```python
from build123d import *

# Parameters (mm, degrees)
EXTRUDE_1_DEPTH                  = 27.5
SKETCH_2_W                       = 5
SKETCH_2_H                       = 21
CUT_EXTRUDE_1_DEPTH              = 3
PATTERN_LINEAR_1_COUNT           = 3
PATTERN_LINEAR_1_PITCH           = 10
PATTERN_LINEAR_2_COPY_1_SKETCH_W = 5
PATTERN_LINEAR_2_COPY_1_SKETCH_H = 21
PATTERN_LINEAR_2_COPY_1_DEPTH    = 3
PATTERN_LINEAR_2_COPY_2_SKETCH_W = 5
PATTERN_LINEAR_2_COPY_2_SKETCH_H = 21
PATTERN_LINEAR_2_COPY_2_DEPTH    = 3
PATTERN_LINEAR_2_COPY_3_SKETCH_W = 5
PATTERN_LINEAR_2_COPY_3_SKETCH_H = 21
PATTERN_LINEAR_2_COPY_3_DEPTH    = 3
PATTERN_LINEAR_2_COPY_4_SKETCH_W = 5
PATTERN_LINEAR_2_COPY_4_SKETCH_H = 21
PATTERN_LINEAR_2_COPY_4_DEPTH    = 3
PATTERN_LINEAR_2_COPY_5_SKETCH_W = 5
PATTERN_LINEAR_2_COPY_5_SKETCH_H = 21
PATTERN_LINEAR_2_COPY_5_DEPTH    = 3
PATTERN_LINEAR_2_COPY_6_SKETCH_W = 5
PATTERN_LINEAR_2_COPY_6_SKETCH_H = 21
PATTERN_LINEAR_2_COPY_6_DEPTH    = 3
CUT_EXTRUDE_2_DEPTH              = 31.504098085
CUT_EXTRUDE_2_DEPTH_BACK         = 55
SKETCH_3_R                       = 2.5
CUT_EXTRUDE_3_DEPTH              = 31.504098085
SKETCH_5_R                       = 4.5
CUT_EXTRUDE_4_DEPTH              = 5.5


with BuildPart() as part:
    # 草图1 → 凸台-拉伸1 (new, symmetric)
    with BuildSketch(Plane(origin=(0, 0, 0), x_dir=(0, 0, -1), z_dir=(1, 0, 0))):
        Polygon((-8, 0), (8, 0), (8, 2.916666667), (10.5, 5), (8, 8), (-8, 8), (-10.5, 5), (-8, 2.916666667), align=None)
    extrude(amount=EXTRUDE_1_DEPTH, both=True)

    # 草图2 → 切除-拉伸1 (cut)
    with BuildSketch(Plane(origin=(0, 8, 0), x_dir=(1, 0, 0), z_dir=(0, 1, 0))):
        Rectangle(SKETCH_2_W, SKETCH_2_H)
    cut_extrude_1 = extrude(amount=-CUT_EXTRUDE_1_DEPTH, mode=Mode.SUBTRACT)

    # 阵列(线性)1: 切除-拉伸1 ×3
    with Locations(*[(i * PATTERN_LINEAR_1_PITCH, 0, 0) for i in range(1, PATTERN_LINEAR_1_COUNT)]):
        add(cut_extrude_1, mode=Mode.SUBTRACT)

    # 阵列(线性)2 copy 1 sketch → 阵列(线性)2 copy 1 (cut)
    with BuildSketch(Plane(origin=(0, 8, 0), x_dir=(1, 0, 0), z_dir=(0, 1, 0))):
        Rectangle(PATTERN_LINEAR_2_COPY_1_SKETCH_W, PATTERN_LINEAR_2_COPY_1_SKETCH_H)
    extrude(amount=-PATTERN_LINEAR_2_COPY_1_DEPTH, mode=Mode.SUBTRACT)

    # 阵列(线性)2 copy 2 sketch → 阵列(线性)2 copy 2 (cut)
    with BuildSketch(Plane(origin=(-10, 8, 0), x_dir=(1, 0, 0), z_dir=(0, 1, 0))):
        Rectangle(PATTERN_LINEAR_2_COPY_2_SKETCH_W, PATTERN_LINEAR_2_COPY_2_SKETCH_H)
    extrude(amount=-PATTERN_LINEAR_2_COPY_2_DEPTH, mode=Mode.SUBTRACT)

    # 阵列(线性)2 copy 3 sketch → 阵列(线性)2 copy 3 (cut)
    with BuildSketch(Plane(origin=(10, 8, 0), x_dir=(1, 0, 0), z_dir=(0, 1, 0))):
        Rectangle(PATTERN_LINEAR_2_COPY_3_SKETCH_W, PATTERN_LINEAR_2_COPY_3_SKETCH_H)
    extrude(amount=-PATTERN_LINEAR_2_COPY_3_DEPTH, mode=Mode.SUBTRACT)

    # 阵列(线性)2 copy 4 sketch → 阵列(线性)2 copy 4 (cut)
    with BuildSketch(Plane(origin=(0, 8, 0), x_dir=(1, 0, 0), z_dir=(0, 1, 0))):
        Rectangle(PATTERN_LINEAR_2_COPY_4_SKETCH_W, PATTERN_LINEAR_2_COPY_4_SKETCH_H)
    extrude(amount=-PATTERN_LINEAR_2_COPY_4_DEPTH, mode=Mode.SUBTRACT)

    # 阵列(线性)2 copy 5 sketch → 阵列(线性)2 copy 5 (cut)
    with BuildSketch(Plane(origin=(-10, 8, 0), x_dir=(1, 0, 0), z_dir=(0, 1, 0))):
        Rectangle(PATTERN_LINEAR_2_COPY_5_SKETCH_W, PATTERN_LINEAR_2_COPY_5_SKETCH_H)
    extrude(amount=-PATTERN_LINEAR_2_COPY_5_DEPTH, mode=Mode.SUBTRACT)

    # 阵列(线性)2 copy 6 sketch → 阵列(线性)2 copy 6 (cut)
    with BuildSketch(Plane(origin=(-20, 8, 0), x_dir=(1, 0, 0), z_dir=(0, 1, 0))):
        Rectangle(PATTERN_LINEAR_2_COPY_6_SKETCH_W, PATTERN_LINEAR_2_COPY_6_SKETCH_H)
    extrude(amount=-PATTERN_LINEAR_2_COPY_6_DEPTH, mode=Mode.SUBTRACT)

    # 草图3 → 切除-拉伸2 (cut, two sides: drawn at the far end of the back side and taken through both)
    with BuildSketch(Plane.XZ.offset(-CUT_EXTRUDE_2_DEPTH_BACK)):
        with Locations(Location((10, 0, 0), (0, 0, 90))):
            Circle(SKETCH_3_R)
        with BuildLine():
            Line((-10, 2.5), (0, 2.5))
            ThreePointArc((0, 2.5), (2.5, 0), (0, -2.5))
            Line((0, -2.5), (-10, -2.5))
            ThreePointArc((-10, -2.5), (-12.5, 0), (-10, 2.5))
        make_face()
    extrude(amount=CUT_EXTRUDE_2_DEPTH + CUT_EXTRUDE_2_DEPTH_BACK, mode=Mode.SUBTRACT)

    # 草图4 → 切除-拉伸3 (cut, symmetric)
    with BuildSketch(Plane.XY):
        Polygon((-27.5, 6.003638962), (-25.5, 8), (-27.5, 8), align=None)
    cut_extrude_3 = extrude(amount=CUT_EXTRUDE_3_DEPTH, both=True, mode=Mode.SUBTRACT)

    # 镜向1: 切除-拉伸3 across plane
    add(cut_extrude_3.mirror(Plane(origin=(0, 0, 0), x_dir=(0, 0, 1), z_dir=(1, 0, 0))), mode=Mode.SUBTRACT)

    # 草图5 → 切除-拉伸4 (cut)
    with BuildSketch(Plane(origin=(0, 8, 0), x_dir=(1, 0, 0), z_dir=(0, 1, 0))):
        with Locations(Location((10, 0, 0), (0, 0, 270))):
            Circle(SKETCH_5_R)
        with BuildLine():
            Line((-10, 4.5), (0, 4.5))
            ThreePointArc((0, 4.5), (4.5, 0), (0, -4.5))
            Line((0, -4.5), (-10, -4.5))
            ThreePointArc((-10, -4.5), (-14.5, 0), (-10, 4.5))
        make_face()
    extrude(amount=-CUT_EXTRUDE_4_DEPTH, mode=Mode.SUBTRACT)


solid = part.part
```
Here's how the part is built. I have some questions about the finished solid (model axes, mm). A direction names the side the tool comes from. Coordinates: 2 decimals unless noted, no trailing zeros. Order: outer loops, then holes, each group sorted by start corner. A loop starts at its lowest first (then second) coordinate and runs counter-clockwise, first axis right, second up. Notation, with made-up numbers: (-36, 87) - (4, 87) arc R35 cw to (4, 122) - close; hole circle Ø8 at (16, 70). An arc over 180 degrees is marked (long way). One line per question, with ' | ' between items. Start each with the question number.
1. I'm going to push flat-ended pins straight in: pin 1 Ø3 at (x, y) = (-4.5, 5.5) entering from +Z; pin 2 Ø3 at (x, y) = (-3.5, 1) entering from -Z; pin 3 Ø0.9 at (x, y) = (0, 2) entering from +Z. Where does each tip first touch, or does it pass through?
2. If we section it at C-C (z = 1.75): Give the number of separate pieces and of enclosed holes in the cut face, and give its area (3 significant figures).
3. If we section it at B-B (y = 3.75): Write out the boundary of the cut face in (x, z).
4. If we section it at D-D (z = -5.25): Write out the boundary of the cut face in (x, y), and give its area (3 significant figures).
5. Please list where these lines run through material, in increasing order: line 1 along X through (y, z) = (0.5, 0); line 2 along X through (y, z) = (5.85, 0); line 3 along X through (y, z) = (5.25, -7). Write a range as [from, to].
6. Which directions (+Z, -Z, +X, -X, +Y, -Y) give clear straight access to the entire face, cutting with the end or side of a thin tool? Please do faces 5 (the flat face through (-5, 2.5, 3)), 6 (the flat face through (5, 8, 0)), 7 (the flat face through (10, 5, 7)).
7. If we mould it in two halves opening along Z, with no side actions, what happens to faces 1 (the cylindrical face through (-12.5, 1.3, -0.1)), 2 (the cylindrical face through (10.198, 4.677, -4.496)), 3 (the flat face through (-22.5, 7, 0)), 4 (the flat face through (0.4, 4, 9.3))? For each: released by +Z, released by -Z, zero draft, split by the parting line, or undercut.
8. If we section it at A-A (x = -9): Write out the boundary of the cut face in (y, z).
Model answer:
1) pin 1: stops at z = 10.5 | pin 2: stops at z = -8 | pin 3: stops at z = 8
2) separate pieces: 3 | enclosed holes: 0 | area: 217 mm²
3) outline: (-27.5, -9) - (27.5, -9) - (27.5, 9) - (-27.5, 9) - close; hole (-10, -4.5) - (0, -4.5) arc R4.5 ccw to (0, 4.5) - (-10, 4.5) arc R4.5 ccw to start; hole circle Ø9 at (10, 0)
4) outline: (-27.5, 0) - (27.5, 0) - (27.5, 6) - (25.5, 8) - (22.5, 8) - (22.5, 5) - (17.5, 5) - (17.5, 8) - (12.5, 8) - (12.5, 5) - (7.5, 5) - (7.5, 8) - (2.5, 8) - (2.5, 5) - (-2.5, 5) - (-2.5, 8) - (-7.5, 8) - (-7.5, 5) - (-12.5, 5) - (-12.5, 8) - (-17.5, 8) - (-17.5, 5) - (-22.5, 5) - (-22.5, 8) - (-25.5, 8) - (-27.5, 6) - close | area: 361 mm²
5) line 1: x = [-27.5, -12.5], [2.5, 7.5], [12.5, 27.5] | line 2: x = [-27.5, -22.5], [-17.5, -14.5], [4.5, 5.5], [14.5, 17.5], [22.5, 27.5] | line 3: x = [-27.5, -22.5], [-17.5, -12.5], [-7.5, -2.5], [2.5, 7.5], [12.5, 17.5], [22.5, 27.5]
6) face 5: +Y | face 6: +Z, -Z, +X, -X, +Y | face 7: +Z, -Z, +Y
7) face 1: undercut | face 2: undercut | face 3: zero draft | face 4: released by +Z
8) outline: (0, -8) - (2.92, -8) - (5, -10.5) - (5, -4.5) - (2.5, -4.5) - (2.5, -2.5) - (0, -2.5) - close; (0, 2.5) - (2.5, 2.5) - (2.5, 4.5) - (5, 4.5) - (5, 10.5) - (2.92, 8) - (0, 8) - close
